Drawing for the job (mm, zero at the part's lowest x, y, z). A direction names the side the tool comes from. Round coordinates to 2 decimals unless told otherwise and drop trailing zeros. Write each loop counter-clockwise with the first axis right and the second up, starting at its lowest first coordinate (ties: lowest second). Pieces come first, ordered by that corner, then holes. Notation, with made-up numbers: (-1, 0) -> (57, 0) arc R19 ccw to (57, 23) -> close; hole circle Ø9 at (11.25, -22.75). An arc over 180 degrees is marked (long way). One line per question, with ' | ' between items.
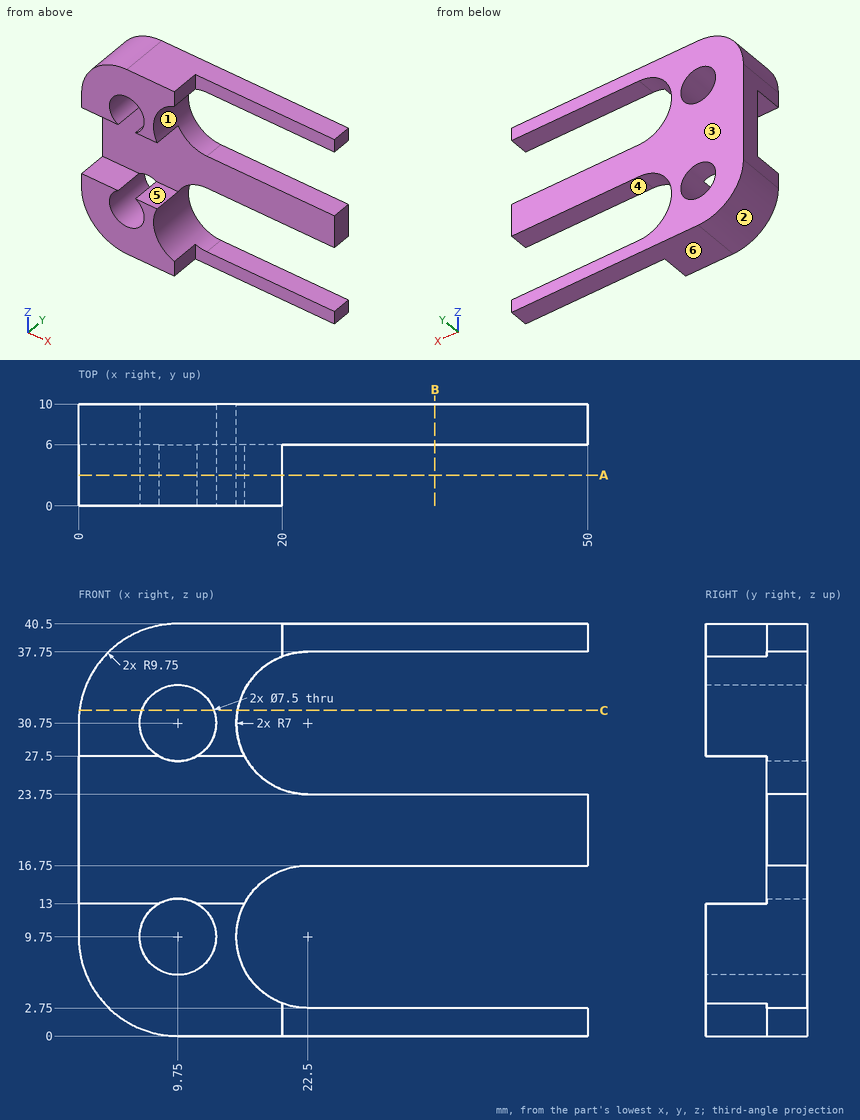
(1) Drop flat-ended pins along their axis: pin 1 (1.6 mm diameter, centred on x = 36.5, z = 1.5, fed in from -Y); pin 2 (8.5 mm diameter, centred on x = 9.75, z = 9.75, fed in from +Y); pin 3 (3.5 mm diameter, centred on y = 3.5, z = 38, fed in from +X); pin 4 (3 mm diameter, centred on x = 30, y = 3.5, fed in from -Z). Give the stop position or say it passes through.
Calculated:
pin 1: y = 6 | pin 2: y = 10 | pin 3: x = 20 | pin 4: through
(2) Slice it at C-C (z = 32). Write the cut outline in (x, y), then the cut area to 3 significant figures.
Calculated:
outline: (0.08, 0) -> (6.21, 0) -> (6.21, 10) -> (0.08, 10) -> close; (13.29, 0) -> (15.61, 0) -> (15.61, 10) -> (13.29, 10) -> close | area: 84.6 mm2
(3) Slice it at A-A (y = 3). Write the cut outline in (x, z).
Calculated:
outline: (0, 9.75) arc R9.75 ccw to (9.75, 0) -> (20, 0) -> (20, 3.21) arc R7 cw to (16.3, 13) -> (11.62, 13) arc R3.75 cw (long way) to (7.88, 13) -> (0, 13) -> close; (0, 27.5) -> (7.88, 27.5) arc R3.75 cw (long way) to (11.62, 27.5) -> (16.3, 27.5) arc R7 cw to (20, 37.29) -> (20, 40.5) -> (9.75, 40.5) arc R9.75 ccw to (0, 30.75) -> close
(4) Mould opens along Z. For the marked faces 1, 2 and 3 say: pulls with the +Z half, pulls with the -Z half, needs draft (parallel to the pull), parting line crosses it, or undercut.
Calculated:
face 1: undercut | face 2: pulls with the -Z half | face 3: needs draft
(5) Wall check: line 1 (Z direction, x = 28.5, y = 9.5); line 2 (X direction, y = 2.75, z = 30.75); line 3 (Z direction, x = 21.5, y = 6.25). Give the ranges that are in metal, low to high. Write a range as from..to.
Calculated:
line 1: 0..2.75, 16.75..23.75, 37.75..40.5 | line 2: 0..6, 13.5..15.5 | line 3: 0..2.82, 16.68..23.82, 37.68..40.5
(6) Slice it at B-B (x = 35). Write the cut outline in (y, z), then the cut area to 3 significant figures.
Calculated:
outline: (6, 0) -> (10, 0) -> (10, 2.75) -> (6, 2.75) -> close; (6, 16.75) -> (10, 16.75) -> (10, 23.75) -> (6, 23.75) -> close; (6, 37.75) -> (10, 37.75) -> (10, 40.5) -> (6, 40.5) -> close | area: 50.0 mm2
(7) 3-axis set-ups, long thin cutter, end or side, ignore diameter. For the marked faces 4, 5 and 6: which of +Z, -Z, +X, -X, +Y, -Y reach the whole face in a straight line?
Calculated:
face 4: +X, +Y, -Y | face 5: +X, -X, -Y | face 6: -Z, +X, -X, +Y, -Y
